Could you check a few things on this model? Use its own coordinates, in mm. Give positions to 0.01 mm unless a question says otherwise; leave off trailing zeros. Order: outer loops, then holes, each group sorted by start corner. A loop starts at its lowest first (then second) coordinate and runs counter-clockwise, first axis right, second up. Notation, with made-up numbers: M 63,-17 L 87,-17 A17 cw 87,14 Z; hole C -27,73.5 d4. An arc over 180 degrees is marked long. Answer in a Markdown table with one row per item. Add a question column.
```python
from build123d import *

# Parameters (mm, degrees)
SKETCH_1_W          = 20
SKETCH_1_H          = 20
EXTRUDE_1_DEPTH     = 130
SKETCH_2_R          = 2.1
CUT_EXTRUDE_1_DEPTH = 132.909059583


with BuildPart() as part:
    # 草图1 → 凸台-拉伸1 (new body)
    with BuildSketch(Plane(origin=(0, 0, 0), x_dir=(1, 0, 0), z_dir=(0, 1, 0))):
        Rectangle(SKETCH_1_W, SKETCH_1_H)
    extrude(amount=EXTRUDE_1_DEPTH)

    # 草图2 → 切除-拉伸1 (cut, through all)
    with BuildSketch(Plane(origin=(10, 0, 0), x_dir=(0, 0, -1), z_dir=(1, 0, 0))):
        with Locations((0, 45)):
            Circle(SKETCH_2_R)
        with Locations((0, 65)):
            Circle(SKETCH_2_R)
        with Locations((0, 85)):
            Circle(SKETCH_2_R)
        with Locations((0, 10)):
            Circle(SKETCH_2_R)
        with Locations((0, 30)):
            Circle(SKETCH_2_R)
        with Locations(Location((0, 100, 0), (0, 0, 180))):
            Circle(SKETCH_2_R)
        with Locations(Location((0, 120, 0), (0, 0, 180))):
            Circle(SKETCH_2_R)
    extrude(amount=-CUT_EXTRUDE_1_DEPTH, mode=Mode.SUBTRACT)


solid = part.part
```
1. If I drill on line 1 along Z through (x, y) = (8, 118.5), over which ranges is the centre line in solid material (lowest first)? Write a range as [from, to].
2. Suppose I cut it at B-B on x = -4.75. List the corners of the cut face in (y, z) for me, plus the area to 3 significant figures.
3. Suppose I cut it at A-A on y = 100. List the corners of the cut face in (x, z) for me.
4. Will these pins go through, and if not, where does the flat tip stop? P1, Ø10, axis at x = -7, z = -6.5, coming from the -Y side; P2, Ø4, axis at y = 10, z = 0, coming from the +X side.
5. Thinking about a two-plate mould opening in Z: for faces 1 (the cylindrical face through (0.14, 12.082, 0.273)), 2 (the flat face through (0, 64, -10)), 3 (the flat face through (10, 64.1, -2.1)), which applies, pulls with the +Z half, pulls with the -Z half, needs draft (parallel to the pull), parting line crosses it, or undercut?
Findings below:
| question | item | result |
|---|---|---|
| 1 | line 1 | [-10, -1.47], [1.47, 10] |
| 2 | outline | M 0,-10 L 130,-10 L 130,10 L 0,10 Z; hole C 10,0 d4.2; hole C 30,0 d4.2; hole C 45,0 d4.2; hole C 65,0 d4.2; hole C 85,0 d4.2; hole C 100,0 d4.2; hole C 120,0 d4.2 |
| 2 | area | 2,500 mm2 |
| 3 | outline | M -10,-10 L 10,-10 L 10,-2.1 L -10,-2.1 Z; M -10,2.1 L 10,2.1 L 10,10 L -10,10 Z |
| 4 | P1 | y = 0 |
| 4 | P2 | through |
| 5 | face 1 | undercut |
| 5 | face 2 | pulls with the -Z half |
| 5 | face 3 | needs draft |
